For this review, use the dimensioned drawing (mm, ordinates from the lowest corner) and the shaded views. A direction names the side the tool comes from. Coordinates: 2 decimals unless noted, no trailing zeros. Order: outer loops, then holes, each group sorted by start corner. A loop starts at its lowest first (then second) coordinate and runs counter-clockwise, first axis right, second up. Notation, with made-up numbers: M 56,-38.75 L 107,-38.75 A27 ccw 107,-22.75 Z; hole C -27.5,29.5 d7. An arc over 180 degrees is marked long. One line per item, written item: value.
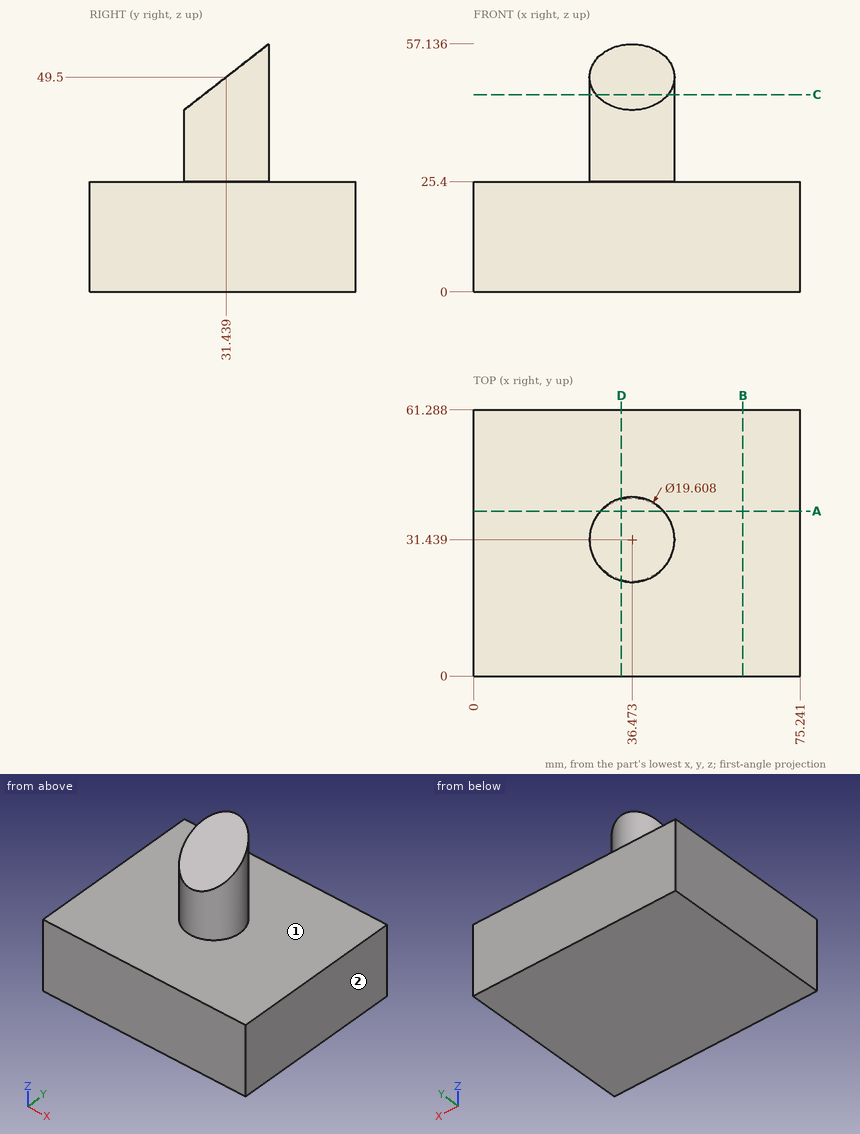
(1) Tool access review of the marked faces 1 and 2: name each direction out of +Z, -Z, +X, -X, +Y, -Y from which nothing blocks a thin tool from reaching the whole face with its end or side.
Geometry results:
face 1: +Z
face 2: +Z, -Z, +X, +Y, -Y
(2) For L1, parallel to Z at x = 16.5, y = 19.5; L2, parallel to Y at x = 30.5, z = 28 (1 decimal); L3, parallel to Y at x = 33, z = 48.5 (1 decimal), list the stretches that pass through material, from the lowest coordinate up.
Geometry results:
L1: z = 0 to 25.4
L2: y = 23.7 to 39.2
L3: y = 30.2 to 40.6
(3) We need section A-A, the plane y = 38. State the section outline as (x, z) points.
Geometry results:
outline: M 0,0 L 75.24,0 L 75.24,25.4 L 43.76,25.4 L 43.76,54.61 L 29.19,54.61 L 29.19,25.4 L 0,25.4 Z
(4) Insertion check: pin 1 Ø4 at (x, y) = (54, 46) entering from +Z; pin 2 Ø12 at (y, z) = (45, 36.5) entering from +X (1 decimal). Each pin has a flat end and moves straight along its axis. Give the tip position at first contact, or say it passes through.
Geometry results:
pin 1: stops at z = 25.4
pin 2: stops at x = 42.7
(5) We need section C-C, the plane z = 45.5. State the section outline as (x, y) points (1 decimal), plus the area to 3 significant figures.
Geometry results:
outline: M 28.1,26.3 L 44.8,26.3 A9.8 ccw long Z
area: 247 mm2
(6) We need section D-D, the plane x = 34. State the section outline as (y, z) points, plus the area to 3 significant figures.
Geometry results:
outline: M 0,0 L 61.29,0 L 61.29,25.4 L 40.93,25.4 L 40.93,56.89 L 21.95,42.11 L 21.95,25.4 L 0,25.4 Z
area: 2,010 mm2
(7) We need section B-B, the plane x = 62. State the section outline as (y, z) points, plus the area to 3 significant figures.
Geometry results:
outline: M 0,0 L 61.29,0 L 61.29,25.4 L 0,25.4 Z
area: 1,560 mm2
